```python
from build123d import *

# Parameters (mm, degrees)
SKETCH1_R                     = 3.175
BOSS_EXTRUDE1_DEPTH           = 3.175
SKETCH2_R                     = 4.444999999999999
BOSS_EXTRUDE2_DEPTH           = 1.27
BOSS_EXTRUDE3_DEPTH           = 1.27
BOSS_EXTRUDE4_DEPTH           = 8.89
BOSS_EXTRUDE4_DEPTH_BACK      = 2.54
SKETCH5_R                     = 3.175
CUT_EXTRUDE1_DEPTH            = 12.7
FILLET1_R                     = 2.54
SKETCH6_W                     = 35.559999999999995
SKETCH6_H                     = 5.08
BOSS_EXTRUDE5_DEPTH           = 8.889999999999999
BOSS_EXTRUDE5_TAPER           = 10.000000000000021
FILLET2_R                     = 1.016
FILLET3_R                     = 2.54
BOSS_EXTRUDE6_DEPTH           = 5.079999999999994
BOSS_EXTRUDE6_TAPER           = 2.000000000000002
FILLET4_R                     = 0.254
FILLET5_R                     = 12.7
BOSS_EXTRUDE7_DEPTH           = 73.66
BOSS_EXTRUDE7_TAPER           = 1.0000000000000022
BOSS_EXTRUDE7_OTHER_WAY_DEPTH = 12.700000000000001
BOSS_EXTRUDE7_OTHER_WAY_TAPER = 1.0000000000000022
FILLET6_R                     = 1.016


with BuildPart() as part:
    # Sketch1 → Boss-Extrude1 (new, symmetric)
    with BuildSketch(Plane(origin=(0, 0, 0), x_dir=(0, 0, -1), z_dir=(1, 0, 0))):
        Circle(SKETCH1_R)
    extrude(amount=BOSS_EXTRUDE1_DEPTH, both=True)

    # Sketch2 → Boss-Extrude2 (add)
    with BuildSketch(Plane(origin=(3.175, 0, 0), x_dir=(0, 0, -1), z_dir=(1, 0, 0))):
        Circle(SKETCH2_R)
    boss_extrude2 = extrude(amount=BOSS_EXTRUDE2_DEPTH)

    # Mirror1: Boss-Extrude2 across plane
    add(boss_extrude2.mirror(Plane(origin=(0, 0, 0), x_dir=(0, 0, 1), z_dir=(1, 0, 0))))

    # Sketch3 → Boss-Extrude3 (add)
    with BuildSketch(Plane(origin=(4.445, 0, 0), x_dir=(0, 0, -1), z_dir=(1, 0, 0))):
        Polygon((-7.3e-16, 1.9049999999999998), (6.349999999999998, 1.9050000000000038), (6.349999999999999, -1.9049999999999998), (4.4e-16, -1.9049999999999998), align=None)
    boss_extrude3 = extrude(amount=-BOSS_EXTRUDE3_DEPTH)

    # Mirror2: Boss-Extrude3 across plane
    add(boss_extrude3.mirror(Plane(origin=(0, 0, 0), x_dir=(0, 0, 1), z_dir=(1, 0, 0))))

    # Sketch4 → Boss-Extrude4 (add, two sides: drawn at the far end of the back side and taken through both)
    with BuildSketch(Plane(origin=(-3.175, 0, 0), x_dir=(0, 0, -1), z_dir=(1, 0, 0)).offset(-BOSS_EXTRUDE4_DEPTH_BACK)):
        with BuildLine():
            Line((1.7374623280944008, 4.773638513592414), (2.1184623280943997, 6.0436385135924136))
            Line((2.1184623280943997, 6.0436385135924136), (5.928462328094399, 6.0436385135924136))
            Line((5.928462328094399, 6.0436385135924136), (9.738462328094398, 8.583638513592414))
            Line((9.738462328094398, 8.583638513592414), (47.838462328094394, 8.583638513592414))
            Line((47.838462328094394, 8.583638513592414), (50.3784623280944, 3.8099999999999996))
            Line((50.3784623280944, 3.8099999999999996), (50.3784623280944, -3.8099999999999996))
            Line((50.3784623280944, -3.8099999999999996), (47.838462328094394, -8.583638513592414))
            Line((47.838462328094394, -8.583638513592414), (9.738462328094398, -8.583638513592414))
            Line((9.738462328094398, -8.583638513592414), (5.928462328094399, -6.0436385135924136))
            Line((5.928462328094399, -6.0436385135924136), (2.1184623280943997, -6.0436385135924136))
            Line((2.1184623280943997, -6.0436385135924136), (1.7374623280944008, -4.773638513592414))
            ThreePointArc((1.7374623280944008, -4.773638513592414), (5.080000000000001, 0), (1.7374623280944008, 4.773638513592414))
        make_face()
    extrude(amount=BOSS_EXTRUDE4_DEPTH + BOSS_EXTRUDE4_DEPTH_BACK)

    # Sketch5 → Cut-Extrude1 (cut)
    with BuildSketch(Plane(origin=(0, 0, -50.3784623280944), x_dir=(-1, 0, 0), z_dir=(0, 0, -1))):
        Circle(SKETCH5_R)
    extrude(amount=-CUT_EXTRUDE1_DEPTH, mode=Mode.SUBTRACT)

    # Fillet1
    fillet1_edges = [part.edges().sort_by_distance(p)[0] for p in [
        (5.715000000000001, -8.583638513592414, -28.788462328094397),
        (-5.715, -8.583638513592414, -28.788462328094397),
        (-5.715, 8.583638513592414, -28.788462328094397),
        (5.715000000000001, 8.583638513592414, -28.788462328094397),
    ]]
    fillet(fillet1_edges, radius=FILLET1_R)

    # Sketch6 → Boss-Extrude5 (add)
    with BuildSketch(Plane(origin=(5.715000000000001, 0, 0), x_dir=(0, 0, -1), z_dir=(1, 0, 0))):
        with Locations((28.7884623280944, 0)):
            Rectangle(SKETCH6_W, SKETCH6_H)
    boss_extrude5 = extrude(amount=BOSS_EXTRUDE5_DEPTH, taper=BOSS_EXTRUDE5_TAPER)

    # Mirror3: Boss-Extrude5 across plane
    add(boss_extrude5.mirror(Plane(origin=(0, 0, 0), x_dir=(0, 0, 1), z_dir=(1, 0, 0))))

    # Fillet2
    fillet2_edges = [part.edges().sort_by_distance(p)[0] for p in [
        (14.605, -1.6e-16, -12.57600918659266),
        (14.605, -0.9724531415017433, -28.788462328094404),
        (14.605, -1.6e-16, -45.00091546959614),
        (14.605, 0.9724531415017431, -28.788462328094397),
        (-14.605, -1.6e-16, -12.57600918659266),
        (-14.605, 0.9724531415017431, -28.788462328094397),
        (-14.605, -1.6e-16, -45.00091546959614),
        (-14.605, -0.9724531415017433, -28.788462328094404),
    ]]
    fillet(fillet2_edges, radius=FILLET2_R)

    # Fillet3
    fillet3_edges = [part.edges().sort_by_distance(p)[0] for p in [
        (5.715000000000001, 0, -11.008462328094403),
        (5.715000000000001, -2.54, -28.7884623280944),
        (5.715000000000001, 0, -46.5684623280944),
        (5.715000000000001, 2.54, -28.7884623280944),
        (-5.715000000000001, 0, -11.008462328094403),
        (-5.715000000000001, -2.54, -28.7884623280944),
        (-5.715000000000001, 0, -46.5684623280944),
        (-5.715000000000001, 2.54, -28.7884623280944),
    ]]
    fillet(fillet3_edges, radius=FILLET3_R)

    # Sketch7 → Boss-Extrude6 (add)
    with BuildSketch(Plane(origin=(0, 8.583638513592414, 0), x_dir=(1, 0, 0), z_dir=(0, 1, 0))):
        Polygon((-1.27, 46.568462328094405), (-2.5399999999999983, 21.168462328094403), (0, 11.0084623280944), (2.5399999999999983, 21.168462328094403), (1.27, 46.568462328094405), align=None)
    boss_extrude6 = extrude(amount=BOSS_EXTRUDE6_DEPTH, taper=BOSS_EXTRUDE6_TAPER)

    # Mirror4: Boss-Extrude6 across plane
    add(boss_extrude6.mirror(Plane.ZX))

    # Fillet4
    fillet4_edges = [part.edges().sort_by_distance(p)[0] for p in [
        (0, 11.123638513592411, -11.3741766617959),
        (0, -11.123638513592411, -11.3741766617959),
    ]]
    fillet(fillet4_edges, radius=FILLET4_R)

    # Fillet5
    # the kernel refuses this fillet: 12.7 mm, written as the material it takes off along each edge
    with BuildSketch(Plane(origin=(26.057756985420163, -13.663638513592407, -46.39106481907633), x_dir=(0, 0.9993908270190958, -0.03489949670250099), z_dir=(-1, 0, 0))) as fillet5_piece_1:
        with BuildLine():
            CenterArc((12.343875700426112, -10.419744967387068), FILLET5_R, 124.86989764584403, 53.130102354155966)
            Line((-0.34838780271640163, -9.976521359265305), (-0.6022330727792515, -9.96765688710287))
            Line((-0.6022330727792515, -9.96765688710287), (-0.2538452700628499, 0.00886447216243524))
            Line((-0.2538452700628499, 0.00886447216243524), (6.6e-16, 0.2539999999999965))
            ThreePointArc((6.6e-16, 0.2539999999999965), (2.5415482425190037, 0.25399999999999656), (4.9378809007302475, 0.2083948993477439))
            Line((4.9378809007302475, 0.2083948993477439), (5.083096485038009, 0))
        make_face()
    extrude(amount=52.11551397084032, mode=Mode.SUBTRACT)
    with BuildSketch(Plane(origin=(26.057756985420163, 13.663638513592407, -46.39106481907633), x_dir=(0, -0.9993908270190958, -0.03489949670250099), z_dir=(-1, 0, 0))) as fillet5_piece_2:
        with BuildLine():
            CenterArc((12.343875700426112, 10.419744967387068), FILLET5_R, 182, 53.13010235415595)
            Line((-0.34838780271640163, 9.976521359265305), (-0.6022330727792515, 9.96765688710287))
            Line((-0.6022330727792515, 9.96765688710287), (-0.2538452700628499, -0.00886447216243524))
            Line((-0.2538452700628499, -0.00886447216243524), (6.6e-16, -0.2539999999999965))
            ThreePointArc((6.6e-16, -0.2539999999999965), (2.5415482425190037, -0.25399999999999656), (4.9378809007302475, -0.2083948993477439))
            Line((4.9378809007302475, -0.2083948993477439), (5.083096485038009, 0))
        make_face()
    extrude(amount=52.11551397084032, mode=Mode.SUBTRACT)

    # Sketch8 → Boss-Extrude7 (add)
    with BuildSketch(Plane(origin=(0, 0, -19.8984623280944), x_dir=(-1, 0, 0), z_dir=(0, 0, -1))):
        Polygon((0, 3.175), (-17.779999999999934, 17.779999999999987), (-3.175, -2e-16), (-17.779999999999934, -17.779999999999987), (0, -3.175), (17.779999999999934, -17.78), (3.175, 0), (17.779999999999934, 17.78), align=None)
    extrude(amount=BOSS_EXTRUDE7_DEPTH, taper=BOSS_EXTRUDE7_TAPER)

    # Sketch8 → Boss-Extrude7 other way (add)
    with BuildSketch(Plane(origin=(0, 0, -19.8984623280944), x_dir=(-1, 0, 0), z_dir=(0, 0, -1))):
        Polygon((0, 3.175), (-17.779999999999934, 17.779999999999987), (-3.175, -2e-16), (-17.779999999999934, -17.779999999999987), (0, -3.175), (17.779999999999934, -17.78), (3.175, 0), (17.779999999999934, 17.78), align=None)
    extrude(amount=-BOSS_EXTRUDE7_OTHER_WAY_DEPTH, taper=BOSS_EXTRUDE7_OTHER_WAY_TAPER)

    # Fillet6
    # the kernel refuses this fillet: 1.016 mm, written as the material it takes off along each edge
    with BuildSketch(Plane(origin=(-20.95567858297953, -20.95567858297961, 5.206103382012049), x_dir=(0.7627077129659504, 0.622551588883571, 0.17523259902424146), z_dir=(0.12452118344129766, 0.12452118344129816, -0.984372363360917))) as fillet6_piece_1:
        with BuildLine():
            CenterArc((FILLET6_R * 10.0405981063, -FILLET6_R), FILLET6_R, 90.0000000000001, 168.62469070380405)
            Line((FILLET6_R * 9.84336321649, -FILLET6_R * 1.98035626088), (0, 0))
            Line((0, 0), (FILLET6_R * 10.0405981063, 3e-17))
        make_face()
    extrude(amount=125.83564515900238, mode=Mode.SUBTRACT)
    with BuildSketch(Plane(origin=(-20.95567858297728, 20.955678582977363, 5.2061033819942395), x_dir=(0.7627077129659501, -0.6225515888835714, 0.17523259902424151), z_dir=(0.12452118344129769, -0.12452118344129823, -0.984372363360917))) as fillet6_piece_2:
        with BuildLine():
            CenterArc((FILLET6_R * 10.0405981063, FILLET6_R), FILLET6_R, 101.37530929619633, 168.62469070380357)
            Line((FILLET6_R * 9.84336321649, FILLET6_R * 1.98035626088), (0, 0))
            Line((0, 0), (FILLET6_R * 10.0405981063, 7e-17))
        make_face()
    extrude(amount=125.8356451589662, mode=Mode.SUBTRACT)
    with BuildSketch(Plane(origin=(20.955678582977644, -20.955678582977715, 5.2061033819972735), x_dir=(-0.6225515888835683, 0.7627077129659525, 0.1752325990242418), z_dir=(-0.1245211834412979, 0.1245211834412984, -0.984372363360917))) as fillet6_piece_3:
        with BuildLine():
            CenterArc((FILLET6_R * 10.0405981063, -FILLET6_R), FILLET6_R, 90, 168.62469070380405)
            Line((FILLET6_R * 9.84336321649, -FILLET6_R * 1.98035626088), (0, 0))
            Line((0, 0), (FILLET6_R * 10.0405981063, 8.1e-16))
        make_face()
    extrude(amount=125.83564515897237, mode=Mode.SUBTRACT)
    with BuildSketch(Plane(origin=(20.955678582978695, 20.95567858297876, 5.2061033820054945), x_dir=(-0.7627077129659505, -0.6225515888835708, 0.17523259902424118), z_dir=(-0.12452118344129749, -0.12452118344129792, -0.984372363360917))) as fillet6_piece_4:
        with BuildLine():
            CenterArc((FILLET6_R * 10.0405981063, -FILLET6_R), FILLET6_R, 90, 168.62469070380394)
            Line((FILLET6_R * 9.84336321649, -FILLET6_R * 1.98035626088), (0, 0))
            Line((0, 0), (FILLET6_R * 10.0405981063, -1.51e-15))
        make_face()
    extrude(amount=125.83564515898904, mode=Mode.SUBTRACT)


solid = part.part
```
For this review, take the finished solid that the model builds, in its own axes (mm). A direction names the side the tool comes from. Round coordinates to 2 decimals unless told otherwise and drop trailing zeros. Write each loop counter-clockwise with the first axis right and the second up, starting at its lowest first coordinate (ties: lowest second). Pieces come first, ordered by that corner, then holes. Notation, with made-up numbers: (77, 60.5) - (95, 60.5) arc R25 cw to (95, 88.5) - close; hole circle Ø8 at (11, 10.25). An arc over 180 degrees is marked (long way). Answer as a JSON object with one key per item and string values.
1. To check wall thickness, follow line 1 along X through (y, z) = (-10, -13.5); line 2 along Y through (x, z) = (-10.25, -16); line 3 along Y through (x, z) = (3, 0) (3 decimals). State the ranges of each line that lie inside material, in increasing order.
Response values:
{"line 1": "x = -11.24 to -8.48, -0.57 to 0.57, 8.48 to 11.24", "line 2": "y = -11.51 to -8.72, -1.74 to 1.74, 8.72 to 11.51", "line 3": "y = -3.175 to 3.175"}
2. We need section B-B on z = -42. Count the separate pieces of the cut face and the enclosed holes in it, then the cut area to 3 significant figures.
Response values:
{"separate pieces": "1", "enclosed holes": "4", "area": "309 mm2"}
3. Draft analysis for pull direction X (two halves, no side actions). For faces 1 (the face through (5.715, 0, -50)), 2 (the face through (7.4, -7.3, -49.9)), 3 (the face through (0.04, -3.1, 0.69)), 4 (the face through (9, 9, -7.198)), state which applies: +X half, -X half, draft (parallel to the pull), parting line (faces both ways), or undercut.
Response values:
{"face 1": "+X half", "face 2": "undercut", "face 3": "undercut", "face 4": "draft"}
4. Tool access review of faces 5 (the face through (-3, 8.584, -29)), 6 (the face through (-5, 0, -50.378)), 7 (the face through (-0.08, 7.3, -7.81)), 8 (the face through (-5.715, 0, -6)): name each direction out of +Z, -Z, +X, -X, +Y, -Y from which nothing blocks a thin tool from reaching the whole face with its end or side.
Response values:
{"face 5": "+Y", "face 6": "-Z, -X", "face 7": "+Z, +Y", "face 8": "+Z, -X"}
5. We need section A-A on z = 0. Give the boundary of the cut face in (x, y) (3 decimals), then the cut area to 3 significant figures.
Response values:
{"outline": "(-4.445, -4.445) - (-3.175, -4.445) - (-3.175, -3.175) - (3.175, -3.175) - (3.175, -4.445) - (4.445, -4.445) - (4.445, 4.445) - (3.175, 4.445) - (3.175, 3.175) - (-3.175, 3.175) - (-3.175, 4.445) - (-4.445, 4.445) - close", "area": "62.9 mm2"}
6. For pin 1 Ø2 at (y, z) = (-7.5, -60.5) entering from +X; pin 2 Ø2.5 at (y, z) = (-2, -1.5) entering from +X (3 decimals); pin 3 Ø1.5 at (y, z) = (-5, -48) entering from -X; pin 4 Ø5.5 at (y, z) = (2, -4) entering from -X (3 decimals), all flat-tipped, find the tip position at first contact; note any pin that passes through.
Response values:
{"pin 1": "passes through", "pin 2": "stops at x = 4.445", "pin 3": "stops at x = -7.26", "pin 4": "stops at x = -5.715"}
